Design review of the part shown in the three views and the two pictorial views. Dimensions are in mm from the part's minimum x, y and z. Round coordinates to 2 decimals unless told otherwise and drop trailing zeros. Order: outer loops, then holes, each group sorted by start corner. A loop starts at its lowest first (then second) coordinate and runs counter-clockwise, first axis right, second up.
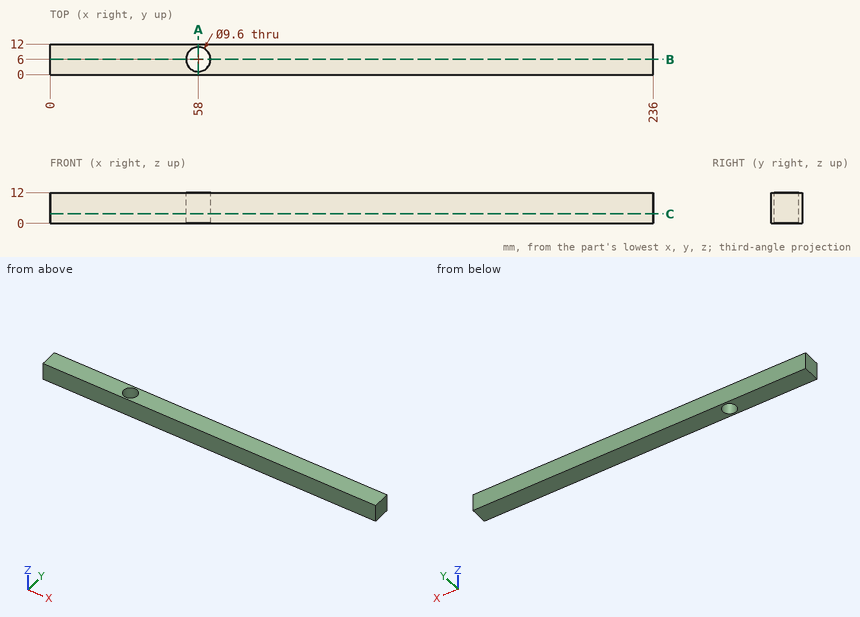
1) Take a section at C-C on z = 3.75. Give the boundary of the cut face in (x, y).
Results:
outline: (0, 0) - (236, 0) - (236, 12) - (0, 12) - close; hole circle Ø9.6 at (58, 6)
2) Take a section at A-A on x = 58. Give the boundary of the cut face in (y, z), plus the area to 3 significant figures.
Results:
outline: (0, 0) - (1.2, 0) - (1.2, 12) - (0, 12) - close; (10.8, 0) - (12, 0) - (12, 12) - (10.8, 12) - close
area: 28.8 mm2
3) To check wall thickness, follow line 1 along X through (y, z) = (6.5, 7.75); line 2 along Y through (x, z) = (58, 7); line 3 along X through (y, z) = (1.75, 5.5). State the ranges of each line that lie inside material, in increasing order.
Results:
line 1: x = 0 to 53.23, 62.77 to 236
line 2: y = 0 to 1.2, 10.8 to 12
line 3: x = 0 to 55.77, 60.23 to 236
4) Clearance check with a flat-ended pin moving along its axis: P1, Ø6, axis at x = 197, z = 4, coming from the -Y side. State where the tip first meets the part, or that it passes through.
Results:
P1: stops at y = 0
5) Take a section at B-B on y = 6. Give the boundary of the cut face in (x, z).
Results:
outline: (0, 0) - (53.2, 0) - (53.2, 12) - (0, 12) - close; (62.8, 0) - (236, 0) - (236, 12) - (62.8, 12) - close
